from build123d import *

# Parameters (mm, degrees)
SKETCH3_R                  = 3.683
CE_00_HOLE_AT_CENTER_DEPTH = 12.7


with BuildPart() as part:
    # Sketch1 → Revolve-Thin1 (revolve)
    with BuildSketch(Plane(origin=(0, 0, 0), x_dir=(0, 0, -1), z_dir=(1, 0, 0)), mode=Mode.PRIVATE) as revolve_thin1_sk:
        with BuildLine():
            ThreePointArc((-3.175, 0), (11.984276071, 46.655454401), (51.671776071, 75.490110981))
            Line((51.671776071, 75.490110981), (94.81101726, 89.506900124))
            ThreePointArc((94.81101726, 89.506900124), (97.98601726, 91.81367265), (99.198759346, 95.546109002))
            Line((99.198759346, 95.546109002), (99.198759346, 114.3))
            Line((99.198759346, 114.3), (97.014359346, 114.3))
            Line((97.014359346, 114.3), (97.014359346, 95.546109002))
            ThreePointArc((97.014359346, 95.546109002), (96.218800538, 93.097630755), (94.136000538, 91.584387978))
            Line((94.136000538, 91.584387978), (50.996759349, 77.567598835))
            ThreePointArc((50.996759349, 77.567598835), (10.217059349, 47.939412506), (-5.3594, 0))
            Line((-5.3594, 0), (-3.175, 0))
        make_face()
    revolve(revolve_thin1_sk.sketch.rotate(Axis((0, 0, -134.341700673), (0, 0, 1)), 90), axis=Axis((0, 0, -134.341700673), (0, 0, 1)))

    # Sketch5 → Cut-Revolve1 (revolve, cut)
    with BuildSketch(Plane(origin=(0, 0, 0), x_dir=(0, 0, -1), z_dir=(1, 0, 0))):
        with BuildLine():
            Line((-8.255, 0), (-23.88640598, 0))
            Line((-23.88640598, 0), (-23.88640598, 127.217845703))
            Line((-23.88640598, 127.217845703), (116.252745686, 127.217845703))
            Line((116.252745686, 127.217845703), (116.252745686, 73.62445992))
            Line((116.252745686, 73.62445992), (88.9, 73.62445992))
            Line((88.9, 73.62445992), (88.9, 92.92772229))
            Line((88.9, 92.92772229), (50.10196974, 80.321478084))
            ThreePointArc((50.10196974, 80.321478084), (7.87446974, 49.641403482), (-8.255, 0))
        make_face()
    revolve(axis=Axis((0, 0, -134.341700673), (0, 0, 1)), mode=Mode.SUBTRACT)

    # Sketch3 → CE-00 Hole at center (cut, symmetric)
    with BuildSketch(Plane.XY):
        with Locations(Location((0, 0, 0), (0, 0, 90))):
            Circle(SKETCH3_R)
    extrude(amount=CE_00_HOLE_AT_CENTER_DEPTH, both=True, mode=Mode.SUBTRACT)


solid = part.part
Geometry check sheet. Reference: the model listing, model coordinates, mm. Give positions to 0.01 mm unless a question says otherwise; leave off trailing zeros. Order: outer loops, then holes, each group sorted by start corner. A loop starts at its lowest first (then second) coordinate and runs counter-clockwise, first axis right, second up.
1) Gauge pin test, flat ends, axial feed: pin 1 (6 mm diameter, centred on y = -28.5, z = -47.5, fed in from -X); pin 2 (5 mm diameter, centred on y = 34, z = -15.5, fed in from -X); pin 3 (1.5 mm diameter, centred on y = 24.5, z = -71, fed in from -X); pin 4 (6 mm diameter, centred on x = 0, y = 0, fed in from +Z). Record the tip position at first contact, or that the pin passes through.
Results are:
pin 1: stops at x = -72.45
pin 2: stops at x = -46.4
pin 3: stops at x = -80.76
pin 4: passes through
2) Cross-section at C-C (z = -64.5). Record the boundary of the cut face in (x, y).
Results are:
outline: circle Ø163.91 at (0, 0); hole circle Ø159.32 at (0, 0)
3) Cross-section at D-D (z = -78). Record the boundary of the cut face in (x, y).
Results are:
outline: circle Ø172.68 at (0, 0); hole circle Ø168.09 at (0, 0)
4) Draft check along Y on faces 1 (the flat face through (86, -20, -88.9)), 2 (the conical face through (10.18, -77.5, -52.84)), 3 (the cylindrical face through (3.267, 1.699, 4.198)). Enter one of: released by +Y, released by -Y, zero draft, split by the parting line, or undercut.
Results are:
face 1: zero draft
face 2: split by the parting line
face 3: undercut
5) Material ranges on probe 1 along X at (y, z) = (-42.5, -32); probe 2 along Y at (x, z) = (-7, -52); probe 3 along X at (y, z) = (-8, -53), recorded low to high.
Results are:
probe 1: x = -53.78 to -50.4, 50.4 to 53.78
probe 2: y = -77.58 to -75.27, 75.27 to 77.58
probe 3: x = -77.81 to -75.5, 75.5 to 77.81
